from build123d import *

# Parameters (mm, degrees)
SZKIC1_R                   = 15
WYCI_GNI_CIE_PROSTE1_DEPTH = 46
SZKIC2_R                   = 14.3
WYCI_GNI_CIE_PROSTE2_DEPTH = 1.5
SZKIC3_R                   = 15
WYCI_GNI_CIE_PROSTE3_DEPTH = 2.1
FAZA1_SIZE                 = 1


with BuildPart() as part:
    # Szkic1 → Wyciągnięcie proste1 (new body)
    with BuildSketch(Plane.XY):
        Circle(SZKIC1_R)
    extrude(amount=WYCI_GNI_CIE_PROSTE1_DEPTH)

    # Szkic2 → Wyciągnięcie proste2 (add)
    with BuildSketch(Plane.XY.offset(46)):
        Circle(SZKIC2_R)
    extrude(amount=WYCI_GNI_CIE_PROSTE2_DEPTH)

    # Szkic3 → Wyciągnięcie proste3 (add)
    with BuildSketch(Plane.XY.offset(47.5)):
        Circle(SZKIC3_R)
    extrude(amount=WYCI_GNI_CIE_PROSTE3_DEPTH)

    # Faza1
    faza1_edges = [part.edges().sort_by_distance(p)[0] for p in [
        (-15, 0, 49.6),
    ]]
    chamfer(faza1_edges, length=FAZA1_SIZE)

    # Odbicie lustrzane1: part across plane


with BuildPart() as part_1:
    add(part.part)
    add(part.part.mirror(Plane(origin=(0, 0, 0), x_dir=(1, 0, 0), z_dir=(0, 0, -1))))


solid = part_1.part
Model file for the job. Use its own axes, mm. A direction names the side the tool comes from. Give positions to 0.01 mm unless a question says otherwise; leave off trailing zeros. Write each loop counter-clockwise with the first axis right and the second up, starting at its lowest first coordinate (ties: lowest second). Pieces come first, ordered by that corner, then holes. Notation, with made-up numbers: (89.25, -10) -> (100.25, -10) arc R12 ccw to (100.25, 1) -> close; hole circle Ø5 at (-31.75, 58.25). An arc over 180 degrees is marked (long way). Write item = value, one per line.
(1) Flat gauge pins, fed straight in: P1, Ø5, axis at x = 9.5, z = -10, coming from the +Y side; P2, Ø10, axis at y = 11.5, z = -5, coming from the +X side; P3, Ø2, axis at x = 9.5, z = -26, coming from the +Y side. Where does each tip first touch, or does it go through?
Determined:
P1 = 13.27
P2 = 13.52
P3 = 12.36
(2) Tool access for faces 1 (the face through (-14.985, 0.66, 0.644)), 2 (the face through (-1.86, 14.18, 46.74)): list every direction of +Z, -Z, +X, -X, +Y, -Y with a clear straight run to the whole face (end or side of a thin tool).
Determined:
face_1 = +Z, -Z
face_2 = none
(3) Slice it at A-A, the plane z = 2. Give the cut face in (x, y), then the cut area to 3 significant figures.
Determined:
outline = circle Ø30 at (0, 0)
area = 707 mm2
(4) Mould opens along Z. For faces 3 (the face through (-14.985, 0.66, -48.042)), 4 (the face through (-1.86, 14.18, -46.74)), 5 (the face through (0, 0, -49.6)) say: released by +Z, released by -Z, zero draft, split by the parting line, or undercut.
Determined:
face_3 = zero draft
face_4 = undercut
face_5 = released by -Z
(5) Probe line 1 along Y through (x, z) = (-0.75, 2); line 2 along X through (y, z) = (-4.5, 39.5); line 3 along Y through (x, z) = (2, 7). List the from-to ranges inside material, lowest first.
Determined:
line_1 = -14.98 to 14.98
line_2 = -14.31 to 14.31
line_3 = -14.87 to 14.87
